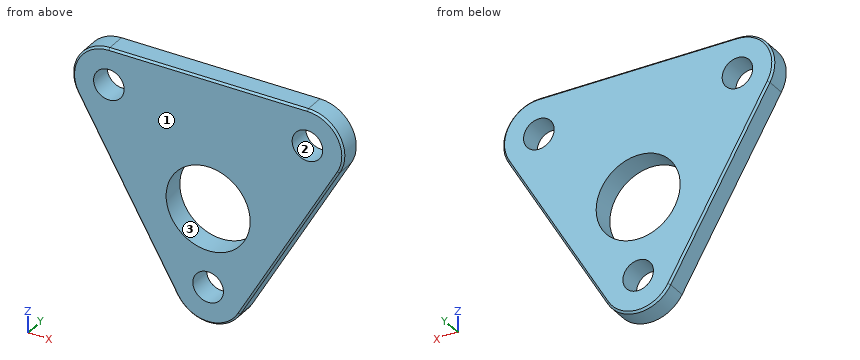
```python
from build123d import *

# Parameters (mm, degrees)
SKETCH_1_R          = 9.5
SKETCH_1_R_2        = 4
EXTRUDE_1_DEPTH     = 6
CHAMFER_1_SIZE      = 0.5
CUT_EXTRUDE_1_REACH = 8
SKETCH_3_R          = 15
SKETCH_4_R          = 15
SKETCH_4_R_2        = 13
EXTRUDE_2_DEPTH     = 6
SKETCH_5_R          = 13
SKETCH_5_R_2        = 11
EXTRUDE_3_DEPTH     = 6


with BuildPart() as part:
    # ｽｹｯﾁ1 → ﾎﾞｽ - 押し出し1 (new body)
    with BuildSketch(Plane(origin=(0, 0, 0), x_dir=(1, 0, 0), z_dir=(0, 1, 0))):
        with BuildLine():
            ThreePointArc((9.5, 30.022213998), (-2.458780928, 20.845918648), (-8.227241336, 34.772213998))
            Line((-8.227241336, 34.772213998), (-34.227241336, -10.261106999))
            ThreePointArc((-34.227241336, -10.261106999), (-23.541219072, -5.834811649), (-16.5, -15.011106999))
            ThreePointArc((-16.5, -15.011106999), (-19.282485579, -21.72862142), (-26, -24.511106999))
            Line((-26, -24.511106999), (26, -24.511106999))
            ThreePointArc((26, -24.511106999), (17.772758664, -10.261106999), (34.227241336, -10.261106999))
            Line((34.227241336, -10.261106999), (8.227241336, 34.772213998))
            ThreePointArc((8.227241336, 34.772213998), (9.17629535, 32.480994926), (9.5, 30.022213998))
        make_face()
        with Locations((-26, -15.011106999)):
            Circle(SKETCH_1_R)
        with Locations((-26, -15.011106999)):
            Circle(SKETCH_1_R_2, mode=Mode.SUBTRACT)
        with Locations((26, -15.011106999)):
            Circle(SKETCH_1_R)
        with Locations((26, -15.011106999)):
            Circle(SKETCH_1_R_2, mode=Mode.SUBTRACT)
        with Locations((0, 30.022213998)):
            Circle(SKETCH_1_R)
        with Locations((0, 30.022213998)):
            Circle(SKETCH_1_R_2, mode=Mode.SUBTRACT)
    extrude(amount=EXTRUDE_1_DEPTH)

    # 面取り1
    chamfer_1_edges = [part.edges().sort_by_distance(p)[0] for p in [
        (-34.227241336, 6, 19.761106999),
        (0, 0, -39.522213998),
        (21.227241336, 0, -12.255553499),
        (34.227241336, 0, 19.761106999),
        (0, 0, 24.511106999),
        (-34.227241336, 0, 19.761106999),
        (-21.227241336, 0, -12.255553499),
        (0, 6, 24.511106999),
        (34.227241336, 6, 19.761106999),
        (21.227241336, 6, -12.255553499),
        (0, 6, -39.522213998),
        (-21.227241336, 6, -12.255553499),
    ]]
    chamfer(chamfer_1_edges, length=CHAMFER_1_SIZE)

    # ｽｹｯﾁ3 → ｶｯﾄ - 押し出し1 (cut, up to next)
    with BuildSketch(Plane.XZ, mode=Mode.PRIVATE) as cut_extrude_1_sk1:
        with Locations((0, -9.5)):
            Circle(SKETCH_3_R)
    cut_extrude_1_tool1 = extrude(cut_extrude_1_sk1.sketch, amount=-CUT_EXTRUDE_1_REACH, mode=Mode.PRIVATE) & part.part
    add(cut_extrude_1_tool1.solids().sort_by_distance((0, 0, -9.5))[0], mode=Mode.SUBTRACT)

    # ｽｹｯﾁ4 → ﾎﾞｽ - 押し出し2 (add)
    with BuildSketch(Plane.XZ):
        with Locations((0, -9.5)):
            Circle(SKETCH_4_R)
        with Locations((0, -9.5)):
            Circle(SKETCH_4_R_2, mode=Mode.SUBTRACT)
    extrude(amount=-EXTRUDE_2_DEPTH)

    # ｽｹｯﾁ5 → ﾎﾞｽ - 押し出し3 (add)
    with BuildSketch(Plane.XZ):
        with Locations((0, -9.5)):
            Circle(SKETCH_5_R)
        with Locations((0, -9.5)):
            Circle(SKETCH_5_R_2, mode=Mode.SUBTRACT)
    extrude(amount=-EXTRUDE_3_DEPTH)


solid = part.part
```
Input: part model. Units: mm. Frame: model coordinates. Face numbers are marked on the shaded views. Give positions to 0.01 mm unless a question says otherwise; leave off trailing zeros. Order: outer loops, then holes, each group sorted by start corner. A loop starts at its lowest first (then second) coordinate and runs counter-clockwise, first axis right, second up. Notation, with made-up numbers: (-34.75, -36.5) - (-13.75, -36.5) arc R38 ccw to (-13.75, 1.5) - close; hole circle Ø3 at (27, -23). An arc over 180 degrees is marked (long way). Use a Markdown table: item, result.
(1) Section query B-B (z = -16). Output: boundary loops of the cut face in (x, y).
Computed values:
| item | result |
|---|---|
| outline | (-19.07, 0.5) - (-18.49, 0) - (-8.87, 0) - (-8.87, 6) - (-18.49, 6) - (-19.07, 5.5) - close; (8.87, 0) - (18.49, 0) - (19.07, 0.5) - (19.07, 5.5) - (18.49, 6) - (8.87, 6) - close |
(2) Pin query (flat end, axial travel): pin 1 (3 mm diameter, centred on y = 3.5, z = -31, fed in from +X); pin 2 (7 mm diameter, centred on x = 0, z = -30.02, fed in from -Y); pin 3 (3 mm diameter, centred on y = 3.5, z = -27, fed in from +X). Return the tip coordinate at first contact, or that it passes through.
Computed values:
| item | result |
|---|---|
| pin 1 | stops at x = 11.27 |
| pin 2 | passes through |
| pin 3 | stops at x = 13.58 |
(3) Section query D-D (x = -10). Output: boundary loops of the cut face in (y, z).
Computed values:
| item | result |
|---|---|
| outline | (0, -30.7) - (0.5, -31.7) - (5.5, -31.7) - (6, -30.7) - (6, -14.08) - (0, -14.08) - close; (0, -4.92) - (6, -4.92) - (6, 24.01) - (5.5, 24.51) - (0.5, 24.51) - (0, 24.01) - close |
(4) Draft query along Z for the marked faces 1, 2 and 3. Return one class per face: released by +Z, released by -Z, zero draft, split by the parting line, or undercut.
Computed values:
| item | result |
|---|---|
| face 1 | zero draft |
| face 2 | undercut |
| face 3 | undercut |
(5) Line query: line 1 (Z direction, x = -1, y = 1.25); line 2 (X direction, y = 1.5, z = -28); line 3 (Z direction, x = -29.5, y = 0.5). Output: solid intervals per line, ascending. Write a range as from..to.
Computed values:
| item | result |
|---|---|
| line 1 | z = -39.47..-33.9, -26.15..-20.45, 1.45..24.51 |
| line 2 | x = -12.14..-3.45, 3.45..12.14 |
| line 3 | z = 2.07..13.07, 16.95..23.84 |
(6) Section query A-A (x = 0). Output: boundary loops of the cut face in (y, z).
Computed values:
| item | result |
|---|---|
| outline | (0, -39.02) - (0.5, -39.52) - (5.5, -39.52) - (6, -39.02) - (6, -34.02) - (0, -34.02) - close; (0, -26.02) - (6, -26.02) - (6, -20.5) - (0, -20.5) - close; (0, 1.5) - (6, 1.5) - (6, 24.01) - (5.5, 24.51) - (0.5, 24.51) - (0, 24.01) - close |
(7) Section query C-C (y = 3.5). Output: boundary loops of the cut face in (x, z), then the cut area to 3 significant figures.
Computed values:
| item | result |
|---|---|
| outline | (-34.23, 10.26) - (-8.23, -34.77) arc R9.5 ccw to (8.23, -34.77) - (34.23, 10.26) arc R9.5 ccw to (26, 24.51) - (-26, 24.51) arc R9.5 ccw to start; hole circle Ø8 at (-26, 15.01); hole circle Ø22 at (0, -9.5); hole circle Ø8 at (0, -30.02); hole circle Ø8 at (26, 15.01) |
| area | 2,410 mm2 |
